Source: three-view drawing plus pictorial views. Frame: mm from the lowest corner of the part. A direction names the side the tool comes from. Round coordinates to 2 decimals unless told otherwise and drop trailing zeros. Order: outer loops, then holes, each group sorted by start corner. A loop starts at its lowest first (then second) coordinate and runs counter-clockwise, first axis right, second up. Notation, with made-up numbers: M 16,73 L 40,73 A29 cw 40,94 Z; hole C 62,-15.75 d7. An arc over 180 degrees is marked long. Return JSON: item names as keys, results as strings. Group by question number.
Q1. Contact query for flat-ended pins moving along their axis: pin 1 (10 mm diameter, centred on y = 34, z = 4.5, fed in from -X); pin 2 (1.9 mm diameter, centred on x = 10, z = 29, fed in from -Y); pin 3 (3.5 mm diameter, centred on x = 10, z = 11, fed in from +Y); pin 4 (8 mm diameter, centred on y = 21.5, z = 13.5, fed in from -X). Output: stop coordinate, or through.
Q2. Access query for the marked faces 1, 2, 3 and 4. Directions: +Z, -Z, +X, -X, +Y, -Y. A direction counts if a zero-diameter tool reaches every point of the face in a straight line with its end or side. Return the directions, or none.
Q3. Cut plane B-B on x = 14.75. Output: boundary loops of the cut face in (y, z).
Q4. Ray query, probe 1 along Z at (x, y) = (10, 2); probe 2 along X at (y, z) = (35.5, 15); probe 3 along X at (y, z) = (6, 11). Return the intervals inside material, ascending.
Q5. Cut plane C-C on y = 6. Output: boundary loops of the cut face in (x, z), and give its area (3 significant figures).
Q6. Cut plane A-A on z = 11. Output: boundary loops of the cut face in (x, y).
Q7. Cut plane D-D on z = 20. Output: boundary loops of the cut face in (x, y).
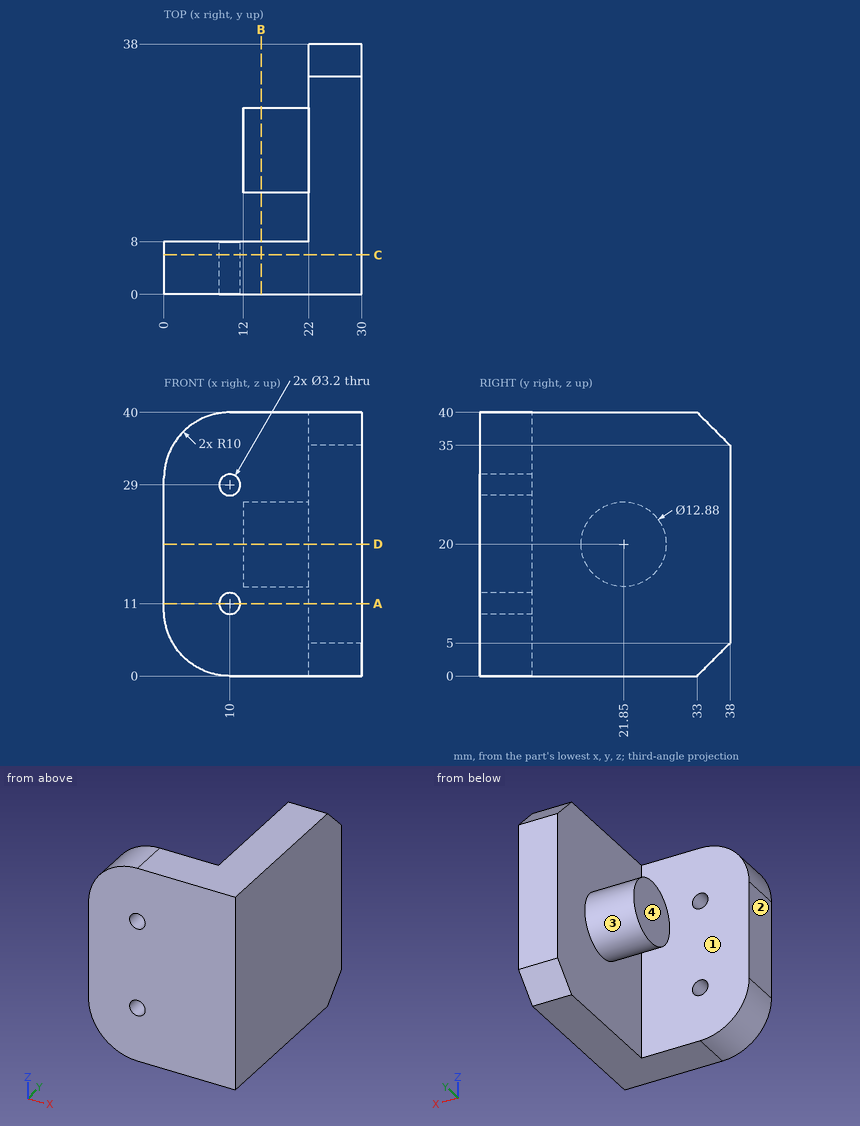
Result sheet:
{
 "1": {"pin 1": "stops at x = 22", "pin 2": "passes through", "pin 3": "stops at y = 8", "pin 4": "stops at x = 12"},
 "2": {"face 1": "+Z, -Z, -X", "face 2": "+Z, -Z, -X, +Y, -Y", "face 3": "-X", "face 4": "+Z, -Z, -X, +Y"},
 "3": {"outline": "M 0,0 L 8,0 L 8,40 L 0,40 Z; C 21.85,20 d12.88"},
 "4": {"probe 1": "z = 0 to 9.4, 12.6 to 27.4, 30.6 to 40", "probe 2": "x = 22 to 30", "probe 3": "x = 0 to 8.4, 11.6 to 30"},
 "5": {"outline": "M 0,10 A10 ccw 10,0 L 30,0 L 30,40 L 10,40 A10 ccw 0,30 Z; hole C 10,11 d3.2; hole C 10,29 d3.2", "area": "1,140 mm²"},
 "6": {"outline": "M 0,0 L 8.4,0 L 8.4,8 L 0,8 Z; M 11.6,0 L 30,0 L 30,38 L 22,38 L 22,8 L 11.6,8 Z"},
 "7": {"outline": "M 0,0 L 30,0 L 30,38 L 22,38 L 22,28.29 L 12,28.29 L 12,15.41 L 22,15.41 L 22,8 L 0,8 Z"}
}
